For this review, take the finished solid that the model builds, in its own axes (mm). Face numbers are marked on the shaded views. A direction names the side the tool comes from. Give positions to 0.01 mm unless a question says otherwise; leave off trailing zeros. Order: outer loops, then holes, each group sorted by start corner. A loop starts at its lowest first (then second) coordinate and runs counter-clockwise, first axis right, second up. Notation, with made-up numbers: (10.5, 30.5) -> (17.5, 30.5) arc R14 ccw to (17.5, 47.5) -> close; hole circle Ø4 at (70, 54.25). An arc over 180 degrees is marked (long way). Return JSON: item names as keys, results as strings. Group by question number.
1) Add section A-A (z = 15.5). Give the boundary of the cut face in (x, y).
2) To check wall thickness, follow line 1 along Z through (x, y) = (-25, -1); line 2 along X through (y, z) = (-3.8, 15); line 3 along X through (y, z) = (-1.2, 6). State the ranges of each line that lie inside material, in increasing order.
3) Add section C-C (y = -0.75). State how many separate pieces and enclosed holes the cut face has, then the cut area to 3 significant figures.
4) Add section B-B (x = -15.5). Give the boundary of the cut face in (y, z).
5) Add section D-D (x = -25). Give the boundary of the cut face in (y, z).
6) The part is to be moulded in two halves that separate along Z. For the marked faces 1, 2, 3 and 4, say which applies: released by +Z, released by -Z, zero draft, split by the parting line, or undercut.
7) Insertion check: P1, Ø2.5, axis at y = -4, z = -6, coming from the -X side; P2, Ø2.5, axis at y = -2.5, z = -5.5, coming from the +X side. Each pin has a flat end and moves straight along its axis. Give the tip position at first contact, or say it passes through.
8) For the marked faces 5, 6 and 7, list the 3-axis set-ups (+Z, -Z, +X, -X, +Y, -Y) from which the entire face can be reached by the end or side of a thin tool; tool diameter is ignored.
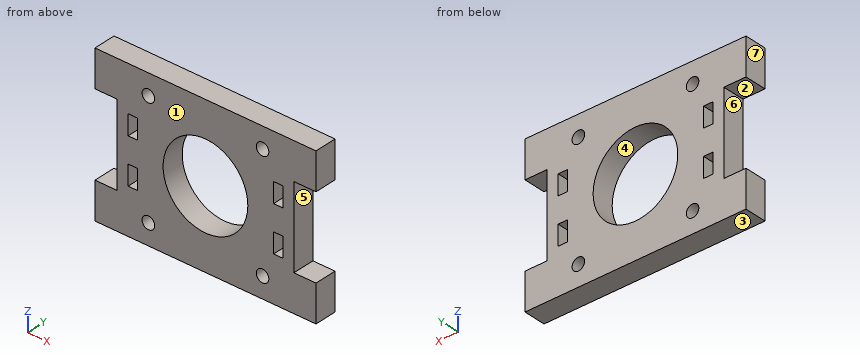
from build123d import *

# Parameters (mm, degrees)
PAD_DEPTH          = 6
SKETCH001_R        = 11.5
POCKET_DEPTH       = 6.001
SKETCH002_W        = 2.5
SKETCH002_H        = 5.4
POCKET001_DEPTH    = 153.314136
SKETCH003_R        = 1.7
POCKET002_DEPTH    = 153.314136
POLARPATTERN_COUNT = 4


with BuildPart() as part:
    # Sketch → Pad (new body)
    with BuildSketch(Plane.XZ):
        Polygon((-30, 21.15), (30, 21.15), (30, 11.15), (24, 11.15), (24, -11.15), (30, -11.15), (30, -21.15), (-30, -21.15), (-30, -11.15), (-24, -11.15), (-24, 11.15), (-30, 11.15), align=None)
    extrude(amount=PAD_DEPTH)

    # Sketch001 (on Face14 of Pad) → Pocket (cut, through all)
    with BuildSketch(Plane.XZ.offset(6)):
        Circle(SKETCH001_R)
    extrude(amount=-POCKET_DEPTH, mode=Mode.SUBTRACT)

    # Sketch002 (on Face5 of Pocket) → Pocket001 (cut, through all)
    with BuildSketch(Plane.XZ.offset(6)):
        with Locations((-19.75, 6.15)):
            Rectangle(SKETCH002_W, SKETCH002_H)
        with Locations((-19.75, -6.15)):
            Rectangle(SKETCH002_W, SKETCH002_H)
    pocket001 = extrude(amount=-POCKET001_DEPTH, mode=Mode.SUBTRACT)

    # Mirrored: Pocket001 across Sketch002 V_Axis
    add(pocket001.mirror(Plane(origin=(0, -6, 0), x_dir=(0, -1, 0), z_dir=(1, 0, 0))), mode=Mode.SUBTRACT)

    # Sketch003 (on Face5 of Mirrored) → Pocket002 (cut, through all)
    with BuildSketch(Plane.XZ.offset(6)):
        with Locations((15.5, 15.5)):
            Circle(SKETCH003_R)
    pocket002 = extrude(amount=-POCKET002_DEPTH, mode=Mode.SUBTRACT)

    # PolarPattern: Pocket002 ×4 about axis
    polarpattern_axis = Axis((0, -6, 0), (0, -1, 0))
    for i in range(1, POLARPATTERN_COUNT):
        add(pocket002.rotate(polarpattern_axis, i * 360 / POLARPATTERN_COUNT), mode=Mode.SUBTRACT)


solid = part.part
Evaluation:
{
 "1": {"outline": "(-30, -6) -> (-17.2, -6) -> (-17.2, 0) -> (-30, 0) -> close; (-13.8, -6) -> (13.8, -6) -> (13.8, 0) -> (-13.8, 0) -> close; (17.2, -6) -> (30, -6) -> (30, 0) -> (17.2, 0) -> close"},
 "2": {"line 1": "-21.15 to -11.15, 11.15 to 21.15", "line 2": "-30 to -17.12, -13.88 to 13.88, 17.12 to 30", "line 3": "-24 to -21, -18.5 to -9.81, 9.81 to 18.5, 21 to 24"},
 "3": {"separate pieces": "1", "enclosed holes": "9", "area": "1,760 mm^2"},
 "4": {"outline": "(-6, -21.15) -> (0, -21.15) -> (0, -17.2) -> (-6, -17.2) -> close; (-6, -13.8) -> (0, -13.8) -> (0, 13.8) -> (-6, 13.8) -> close; (-6, 17.2) -> (0, 17.2) -> (0, 21.15) -> (-6, 21.15) -> close"},
 "5": {"outline": "(-6, -21.15) -> (0, -21.15) -> (0, -11.15) -> (-6, -11.15) -> close; (-6, 11.15) -> (0, 11.15) -> (0, 21.15) -> (-6, 21.15) -> close"},
 "6": {"face 1": "zero draft", "face 2": "undercut", "face 3": "released by -Z", "face 4": "undercut"},
 "7": {"P1": "x = -24", "P2": "x = 24"},
 "8": {"face 5": "+X, +Y, -Y", "face 6": "-X, +Y, -Y", "face 7": "+Z, -Z, -X, +Y, -Y"}
}
